Print and shaded views of the part. All mm, measured from the part's lowest x, y and z. A direction names the side the tool comes from. Coordinates: 2 decimals unless noted, no trailing zeros. Order: outer loops, then holes, each group sorted by start corner. A loop starts at its lowest first (then second) coordinate and runs counter-clockwise, first axis right, second up. Notation, with made-up numbers: (81.5, 26.25) - (116.5, 26.25) arc R19 cw to (116.5, 50.25) - close; hole circle Ø9 at (3.5, 70.5). An arc over 180 degrees is marked (long way). Write each question's results on one line, items separated by ' | '.
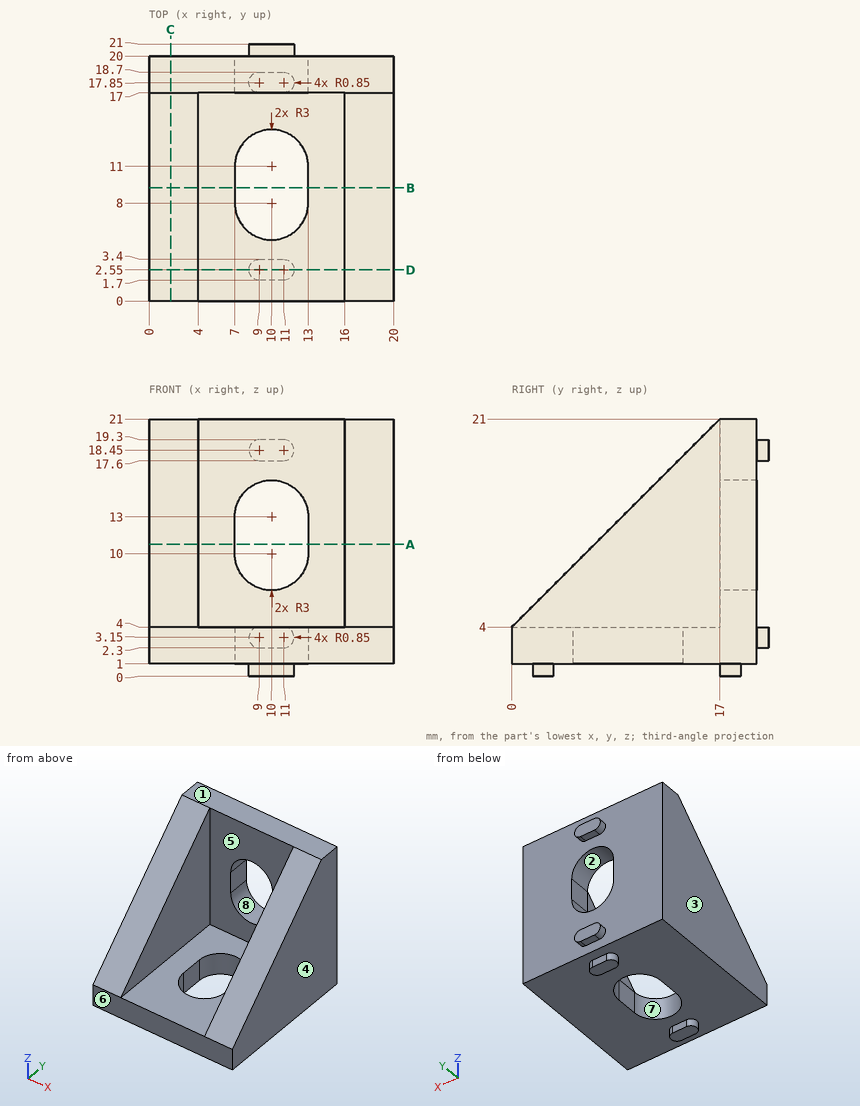
1. Band-saw the part on C-C on x = 1.75. Give the cut face in (y, z).
Solved:
outline: (0, 1) - (20, 1) - (20, 21) - (17, 21) - (0, 4) - close
2. Band-saw the part on B-B on y = 9.25. Give the cut face in (x, z).
Solved:
outline: (0, 1) - (7, 1) - (7, 4) - (4, 4) - (4, 13.25) - (0, 13.25) - close; (13, 1) - (20, 1) - (20, 13.25) - (16, 13.25) - (16, 4) - (13, 4) - close
3. Two-plate mould, pull along X, no slides. Class the marked faces 1, 2 and 3: +X half, -X half, draft (parallel to the pull), parting line (faces both ways), or undercut.
Solved:
face 1: draft | face 2: undercut | face 3: -X half
4. Band-saw the part on D-D on y = 2.55. Give the cut face in (x, z), then the cut area to 3 significant figures.
Solved:
outline: (0, 1) - (8.15, 1) - (8.15, 0) - (11.85, 0) - (11.85, 1) - (20, 1) - (20, 6.55) - (16, 6.55) - (16, 4) - (4, 4) - (4, 6.55) - (0, 6.55) - close | area: 84.1 mm2
5. Band-saw the part on A-A on z = 10.75. Give the cut face in (x, y), then the cut area to 3 significant figures.
Solved:
outline: (0, 6.75) - (4, 6.75) - (4, 17) - (7, 17) - (7, 20) - (0, 20) - close; (13, 17) - (16, 17) - (16, 6.75) - (20, 6.75) - (20, 20) - (13, 20) - close | area: 124 mm2
6. Drop flat-ended pins along their axis: pin 1 Ø3 at (x, z) = (9, 7.5) entering from +Y; pin 2 Ø0.5 at (x, y) = (9.5, 20.5) entering from +Z; pin 3 Ø0.5 at (x, z) = (10, 0.5) entering from +Y. Give the stop position or say it passes through.
Solved:
pin 1: stops at y = 20 | pin 2: stops at z = 19.3 | pin 3: stops at y = 18.7
7. Tool access for the marked faces 4, 5, 6, 7 and 8: list every direction of +Z, -Z, +X, -X, +Y, -Y with a clear straight run to the whole face (end or side of a thin tool).
Solved:
face 4: +Z, -Z, +X, +Y, -Y | face 5: +Z, -Y | face 6: +Z, -Z, +X, -X, -Y | face 7: +Z, -Z | face 8: +Y, -Y
8. Probe line 1 (X direction, y = 9.5, z = 3.5); line 2 (X direction, y = 16.5, z = 17.75); line 3 (Z direction, x = 10, y = 1). List the from-to ranges inside material, lowest first.
Solved:
line 1: x = 0 to 7, 13 to 20 | line 2: x = 0 to 4, 16 to 20 | line 3: z = 1 to 4
